Can you work these out from the model? Positions are in its coordinate system, mm. A direction names the side the tool comes from. Give positions to 0.01 mm unless a question says otherwise; leave off trailing zeros. Loops run counter-clockwise (first coordinate to the right, second up) from the corner with the lowest first, then second, coordinate; pieces in that order, holes last. Notation, with made-up numbers: M -15.75,29.25 L 35.25,29.25 A26 cw 35.25,60.25 Z; hole C 44.5,12 d2. An arc over 180 degrees is marked long. Use CSV: the item, a comma, the result in double quotes.
from build123d import *

# Parameters (mm, degrees)
SKETCH5_W          = 4
SKETCH5_H          = 5
CUT_EXTRUDE1_DEPTH = 106.250863209
CIRPATTERN1_START  = -2.5
CIRPATTERN1_DEPTH  = 5


# Read off the part's stored shape, not the designer's step: CirPattern1
with BuildPart() as part:
    # Sketch4 → Revolve1 (revolve)
    with BuildSketch(Plane(origin=(0, 0, 0), x_dir=(0, 0, -1), z_dir=(1, 0, 0))):
        with BuildLine():
            ThreePointArc((-70, -13), (-66.146279116, 0), (-70, 13))
            ThreePointArc((-70, 13), (-73.853720884, 0), (-70, -13))
        make_face()
    revolve(axis=Axis((0, 13, 0), (0, -1, 0)))

    # Sketch5 → Cut-Extrude1 (cut, symmetric)
    with BuildSketch(Plane.XY):
        with Locations((-73.853720884, 0)):
            Rectangle(SKETCH5_W, SKETCH5_H)
    extrude(amount=CUT_EXTRUDE1_DEPTH, both=True, mode=Mode.SUBTRACT)

    # CirPattern1 outline → CirPattern1 (cut)
    with BuildSketch(Plane(origin=(0, 0, 0), x_dir=(1, 0, 0), z_dir=(0, 1, 0)).offset(CIRPATTERN1_START)):
        Polygon((-57.497286734, -44.119219847), (-66.957008549, -27.734501037), (-71.853720884, -9.459721815), (-71.853720884, -75), (75, -75), (75, 75), (-71.853720884, 75), (-71.853720884, 9.459721815), (-66.957008549, 27.734501037), (-57.497286734, 44.119219847), (-44.119219847, 57.497286734), (-27.734501037, 66.957008549), (-9.459721815, 71.853720884), (9.459721815, 71.853720884), (27.734501037, 66.957008549), (44.119219847, 57.497286734), (57.497286734, 44.119219847), (66.957008549, 27.734501037), (71.853720884, 9.459721815), (71.853720884, -9.459721815), (66.957008549, -27.734501037), (57.497286734, -44.119219847), (44.119219847, -57.497286734), (27.734501037, -66.957008549), (9.459721815, -71.853720884), (-9.459721815, -71.853720884), (-27.734501037, -66.957008549), (-44.119219847, -57.497286734), align=None)
    extrude(amount=CIRPATTERN1_DEPTH, mode=Mode.SUBTRACT)


solid = part.part
Q1. I'm going to push flat-ended pins straight in: P1, Ø4, axis at x = -2, y = 9.5, coming from the -Z side; P2, Ø8, axis at x = 2.5, y = -10, coming from the -Z side; P3, Ø2.5, axis at x = -0.5, y = 0.5, coming from the -Z side; P4, Ø8, axis at x = -54.5, z = -58.5, coming from the -Y side. Where does each tip first touch, or does it pass through?
Model answer:
P1,"z = -72.62"
P2,"z = -73.05"
P3,"z = -71.85"
P4,"through"
Q2. I want a section at A-A, the plane z = 0. Please give me the cut outline in (x, y), then the cut area to 3 significant figures.
Model answer:
outline,"M -73.72,-2.5 A23.85 ccw -70,-13 A23.85 ccw -70,13 A23.85 ccw -73.72,2.5 L -71.85,2.5 L -71.85,-2.5 Z; M 70,-13 A23.85 ccw 73.72,-2.5 L 71.85,-2.5 L 71.85,2.5 L 73.72,2.5 A23.85 ccw 70,13 A23.85 ccw Z"
area,"252 mm2"
Q3. I want a section at B-B, the plane y = 0. Please give me the cut outline in (x, z), then the cut area to 3 significant figures.
Model answer:
outline,"M -71.85,-9.46 L -66.96,-27.73 L -57.5,-44.12 L -44.12,-57.5 L -27.73,-66.96 L -9.46,-71.85 L 9.46,-71.85 L 27.73,-66.96 L 44.12,-57.5 L 57.5,-44.12 L 66.96,-27.73 L 71.85,-9.46 L 71.85,9.46 L 66.96,27.73 L 57.5,44.12 L 44.12,57.5 L 27.73,66.96 L 9.46,71.85 L -9.46,71.85 L -27.73,66.96 L -44.12,57.5 L -57.5,44.12 L -66.96,27.73 L -71.85,9.46 Z; hole C 0,0 d132.29"
area,"2,570 mm2"
Q4. I want a section at C-C, the plane y = -9.5. Please give me the cut outline in (x, z).
Model answer:
outline,"C 0,0 d143.76; hole C 0,0 d136.24"
Q5. For faces 1 (the flat face through (18.73, -0.04, 69.37)), 2 (the flat face through (71.854, 0, 0)), 3 (the flat face through (-36.04, -0.04, -62.16)), 4 (the flat face through (-71.854, 0, 0)), which set-ups out of +Z, -Z, +X, -X, +Y, -Y let a thin tool reach every point of the face, with its end or its side?
Model answer:
face 1,"+Z, +X"
face 2,"+Z, -Z, +X"
face 3,"-Z, -X"
face 4,"+Z, -Z, -X"
Q6. Please list where these lines run through material, in increasing order: L1, parallel to X at y = -10.5, z = -28.5; L2, parallel to Z at x = -54.5, y = -5.25; L3, parallel to Z at x = 14, y = 2.25. Write a range as from..to.
Model answer:
L1,"-65.49..-62.38, 62.38..65.49"
L2,"-48.97..-38.51, 38.51..48.97"
L3,"-70.64..-64.76, 64.76..70.64"
Q7. I want a section at D-D, the plane y = 9. Please give me the cut outline in (x, z), then the cut area to 3 significant figures.
Model answer:
outline,"C 0,0 d144.18; hole C 0,0 d135.82"
area,"1,840 mm2"
